Autodesk Fusion 360 part; units mm, degrees
sketch "Sketch1" plane through (0, 0, 0) normal (0, 0, 1) x (1, 0, 0)
  line L0 (0, 0) -> (103.5, 0)
  line L1 (103.5, 0) -> (103.5, 47)
  line L2 (103.5, 47) -> (0, 47)
  line L3 (0, 47) -> (0, 0)
  line L4 (-6.5, -6.5) -> (110, -6.5)
  line L5 (110, -6.5) -> (110, 53.5)
  line L6 (110, 53.5) -> (-6.5, 53.5)
  line L7 (-6.5, 53.5) -> (-6.5, -6.5)
  line L8 (0, 0) -> (7.051, 0) construction
  circle A0 centre (4.8, 5) radius 1.3
  circle A1 centre (5, 41.9) radius 1.3
  circle A2 centre (98.5, 42.2) radius 1.3
  circle A3 centre (98.5, 5) radius 1.3
  circle A4 centre (-0.5, -0.5) radius 4.25
  circle A5 centre (104, -0.5) radius 4.25
  circle A6 centre (-0.5, 47.5) radius 4.25
  circle A7 centre (104, 47.5) radius 4.25
  line L9 (6.5, 6.5) -> (97, 6.5)
  line L10 (97, 6.5) -> (97, 40.5)
  line L11 (97, 40.5) -> (6.5, 40.5)
  line L12 (6.5, 40.5) -> (6.5, 6.5)
  dimension "d1" = 103.5
  dimension "d2" = 47
  dimension "d3" = 6.5
  dimension "d6" = 2.6
  dimension "d7" = 2.6
  dimension "d9" = 2.6
  dimension "d11" = 2.6
  dimension "d20" = 5
  dimension "d21" = 5.1
  dimension "d22" = 5
  dimension "d23" = 4.8
  dimension "d24" = 5
  dimension "d25" = 5
  dimension "d26" = 4.8
  dimension "d27" = 5
  dimension "d30" = 8.5
  dimension "d31" = 8.5
  dimension "d32" = 8.5
  dimension "d33" = 8.5
  dimension "d34" = 6
  dimension "d36" = 6
  dimension "d37" = 6
  dimension "d38" = 6
  dimension "d39" = 6
  dimension "d40" = 6
  dimension "d41" = 6
  dimension "d42" = 6
  dimension "d45" = -6.5
extrude "Extrude1" add sketch "Sketch1" along normal blind 10 contours L0 L3 A4 | L0 L3 A4 | L0 L1 L2 L3 A4 A5 A6 A7 | L0 L1 A5 | L0 L1 A5 | L2 L3 A6 | L2 L3 A6 | L1 L2 A7 | L1 L2 A7 | L4 L5 L6 L7 | L9 L10 L11 L12
extrude "Extrude2" add sketch "Sketch1" along normal blind 14 contours L0 L3 A4 | L0 L1 A5 | L2 L3 A6 | L1 L2 A7 | L4 L5 L6 L7 picked at (-2.4457, -2.2102) picked at (105.7715, -2.3893) picked at (-2.4457, 49.2102) picked at (105.7715, 49.3893)
extrude "Extrusion4" add sketch "Sketch1" along normal blind 12.2 contours L0 L3 A4 | L0 L1 L2 L3 A4 A5 A6 A7 | L0 L1 A5 | L2 L3 A6 | L1 L2 A7 picked at (-2.4457, -2.2102) picked at (105.7715, -2.3893) picked at (1.6646, 45.3354) picked at (105.7715, 49.3893)
fillet "Fillet1" radius 5 4 edges at (-6.5, 53.5, 7) (110, 53.5, 7) (110, -6.5, 7) (-6.5, -6.5, 7)
extrude "Extrusion3" cut sketch "Sketch1" along normal blind 3.2 contours L0 L3 A4 | L0 L3 A4 | L0 L1 A5 | L0 L1 A5 | L2 L3 A6 | L2 L3 A6 | L1 L2 A7 | L1 L2 A7
Build history of the part. All positions in model axes, mm. A direction names the side the tool comes from. Coordinates: 2 decimals unless noted, no trailing zeros. Order: outer loops, then holes, each group sorted by start corner. A loop starts at its lowest first (then second) coordinate and runs counter-clockwise, first axis right, second up. Notation, with made-up numbers: (15.25, 16) -> (48.25, 16) arc R27 ccw to (48.25, 55) -> close; hole circle Ø3 at (-17.75, 82.25). An arc over 180 degrees is marked (long way). Answer in a Markdown table with one row per item. Add a question column.
Q1. Band-saw the part on B-B, the plane x = 98.5. List the corners of the cut face in (y, z), then the cut area to 3 significant figures.
Q2. Drop flat-ended pins along their axis: pin 1 (17 mm diameter, centred on x = 44, y = 17, fed in from +Z); pin 2 (5 mm diameter, centred on x = 104, y = 47.5, fed in from -Z); pin 3 (2 mm diameter, centred on x = 5, y = 41.9, fed in from +Z). Give the stop position or say it passes through.
Q3. Band-saw the part on A-A, the plane z = 2. Give the number of separate pieces and of enclosed holes in the cut face, then the cut area to 3 significant figures.
Q4. Band-saw the part on D-D, the plane y = 30. List the corners of the cut face in (x, z).
Q5. Which spindle directions (+Z, -Z, +X, -X, +Y, -Y) get a long thin tool onto all of the face, cutting with end or side? Do faces 1 (the face through (104, 0, 3.2)), 2 (the face through (51, 0, 13)), 3 (the face through (99.7, 42.7, 6)). Say none if no direction does.
Q6. Wall check: line 1 along X through (y, z) = (47.5, 1.15); line 2 along Y through (x, z) = (-0.5, 1.7); line 3 along Y through (x, z) = (70.5, 13.25). Give the ranges that are in metal, low to high. Write a range as [from, to].
Q7. Band-saw the part on C-C, the plane y = 5. List the corners of the cut face in (x, z), then the cut area to 3 significant figures.
Q8. Mould opens along Y. For faces 4 (the face through (-1.42, 51.65, 1.58)), 5 (the face through (51, -6.5, 7)), 6 (the face through (-6.5, 24, 7)) say: +Y half, -Y half, draft (parallel to the pull), parting line (faces both ways), or undercut.
Answers follow:
| question | item | result |
|---|---|---|
| 1 | outline | (-6.5, 0) -> (3.7, 0) -> (3.7, 12.2) -> (0, 12.2) -> (0, 14) -> (-6.5, 14) -> close; (6.3, 0) -> (40.9, 0) -> (40.9, 12.2) -> (6.3, 12.2) -> close; (43.5, 0) -> (53.5, 0) -> (53.5, 14) -> (47, 14) -> (47, 12.2) -> (43.5, 12.2) -> close |
| 1 | area | 692 mm^2 |
| 2 | pin 1 | z = 10 |
| 2 | pin 2 | z = 3.2 |
| 2 | pin 3 | through |
| 3 | separate pieces | 1 |
| 3 | enclosed holes | 8 |
| 3 | area | 6,720 mm^2 |
| 4 | outline | (-6.5, 0) -> (110, 0) -> (110, 14) -> (103.5, 14) -> (103.5, 12.2) -> (97, 12.2) -> (97, 10) -> (6.5, 10) -> (6.5, 12.2) -> (0, 12.2) -> (0, 14) -> (-6.5, 14) -> close |
| 5 | face 1 | -Z |
| 5 | face 2 | +Z |
| 5 | face 3 | +Z, -Z |
| 6 | line 1 | [-6.5, -4.75], [3.75, 99.75], [108.25, 110] |
| 6 | line 2 | [-6.5, -4.75], [3.75, 43.25], [51.75, 53.5] |
| 6 | line 3 | [-6.5, 0], [47, 53.5] |
| 7 | outline | (-6.5, 0) -> (3.5, 0) -> (3.5, 12.2) -> (0, 12.2) -> (0, 14) -> (-6.5, 14) -> close; (6.1, 0) -> (97.2, 0) -> (97.2, 12.2) -> (6.1, 12.2) -> close; (99.8, 0) -> (110, 0) -> (110, 14) -> (103.5, 14) -> (103.5, 12.2) -> (99.8, 12.2) -> close |
| 7 | area | 1,380 mm^2 |
| 8 | face 4 | undercut |
| 8 | face 5 | -Y half |
| 8 | face 6 | draft |
